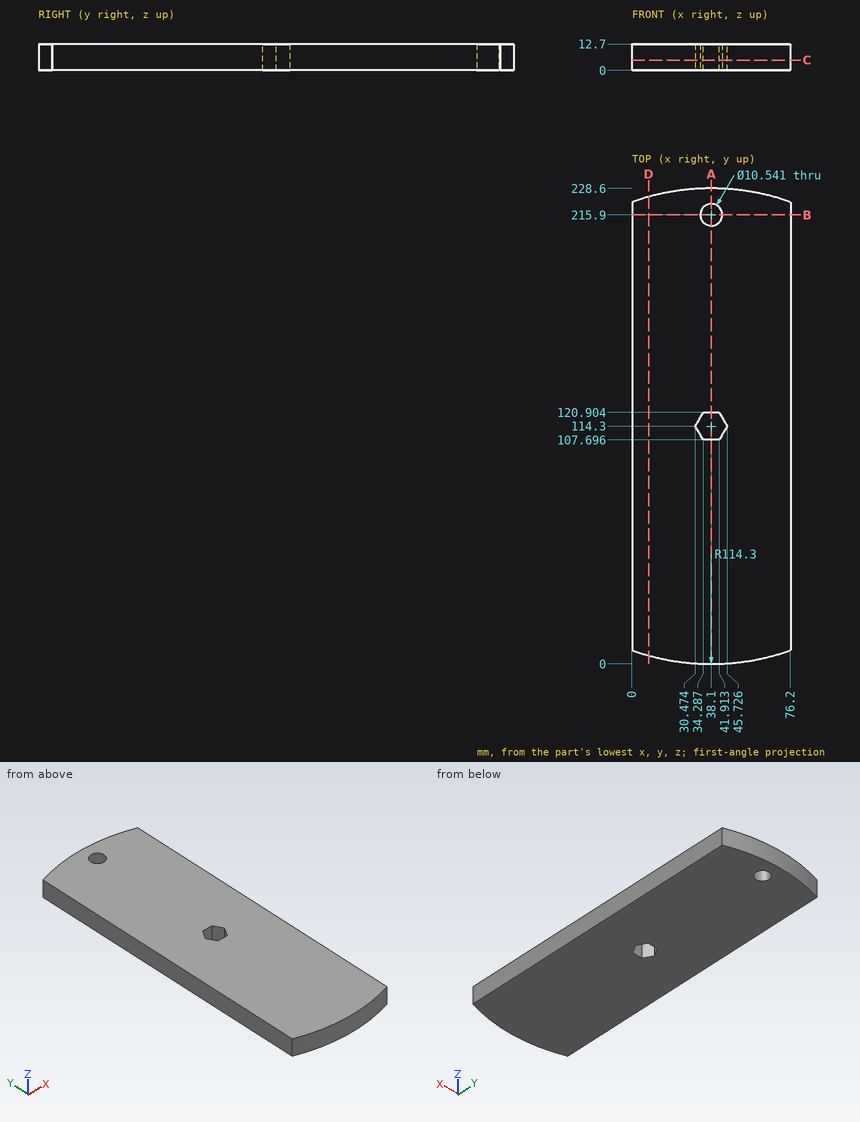
Input: dimensioned drawing with shaded views. Units: mm. Origin: part minimum x, y, z. Coordinates: 2 decimals unless noted, no trailing zeros. Order: outer loops, then holes, each group sorted by start corner. A loop starts at its lowest first (then second) coordinate and runs counter-clockwise, first axis right, second up. Notation, with made-up numbers: M 18.25,58.25 L 42.25,58.25 A18 cw 42.25,68.25 Z; hole C -0.5,64 d8. An arc over 180 degrees is marked long. Answer as CSV lines item,"result".
Q1. Section C-C on z = 5. Return the cut outline in (x, y) (1 decimal).
Answers:
outline,"M 0,6.5 A114.3 ccw 76.2,6.5 L 76.2,222.1 A114.3 ccw 0,222.1 Z; hole M 30.5,114.3 L 34.3,107.7 L 41.9,107.7 L 45.7,114.3 L 41.9,120.9 L 34.3,120.9 Z; hole C 38.1,215.9 d10.5"
Q2. Section A-A on x = 38.1. Return the cut outline in (y, z).
Answers:
outline,"M 0,0 L 107.7,0 L 107.7,12.7 L 0,12.7 Z; M 120.9,0 L 210.63,0 L 210.63,12.7 L 120.9,12.7 Z; M 221.17,0 L 228.6,0 L 228.6,12.7 L 221.17,12.7 Z"
Q3. Section D-D on x = 8. Return the cut outline in (y, z) (1 decimal).
Answers:
outline,"M 4,0 L 224.6,0 L 224.6,12.7 L 4,12.7 Z"
Q4. First-contact query: P1, Ø4, axis at x = 45.5, z = 9.5, coming from the -Y side; P2, Ø8.5, axis at x = 38.1, y = 215.9, coming from the -Z side; P3, Ø3, axis at x = 9.5, z = 7.5, coming from the +Y side. Flat tips, straight axial feed; report the tip coordinate or a pass-through.
Answers:
P1,"stops at y = 0.13"
P2,"passes through"
P3,"stops at y = 225.34"
Q5. Section B-B on y = 215.9. Return the cut outline in (x, z).
Answers:
outline,"M 0,0 L 32.83,0 L 32.83,12.7 L 0,12.7 Z; M 43.37,0 L 76.2,0 L 76.2,12.7 L 43.37,12.7 Z"
Q6. Line query: probe 1 along Y at (x, z) = (38.1, 4.5); probe 2 along X at (y, z) = (215.9, 4.5); probe 3 along Y at (x, z) = (33.5, 12) (1 decimal). Output: solid intervals per line, ascending. Write a range as [from, to].
Answers:
probe 1,"y = [0, 107.7], [120.9, 210.63], [221.17, 228.6]"
probe 2,"x = [0, 32.83], [43.37, 76.2]"
probe 3,"y = [0.1, 109.1], [119.5, 213.3], [218.5, 228.5]"
